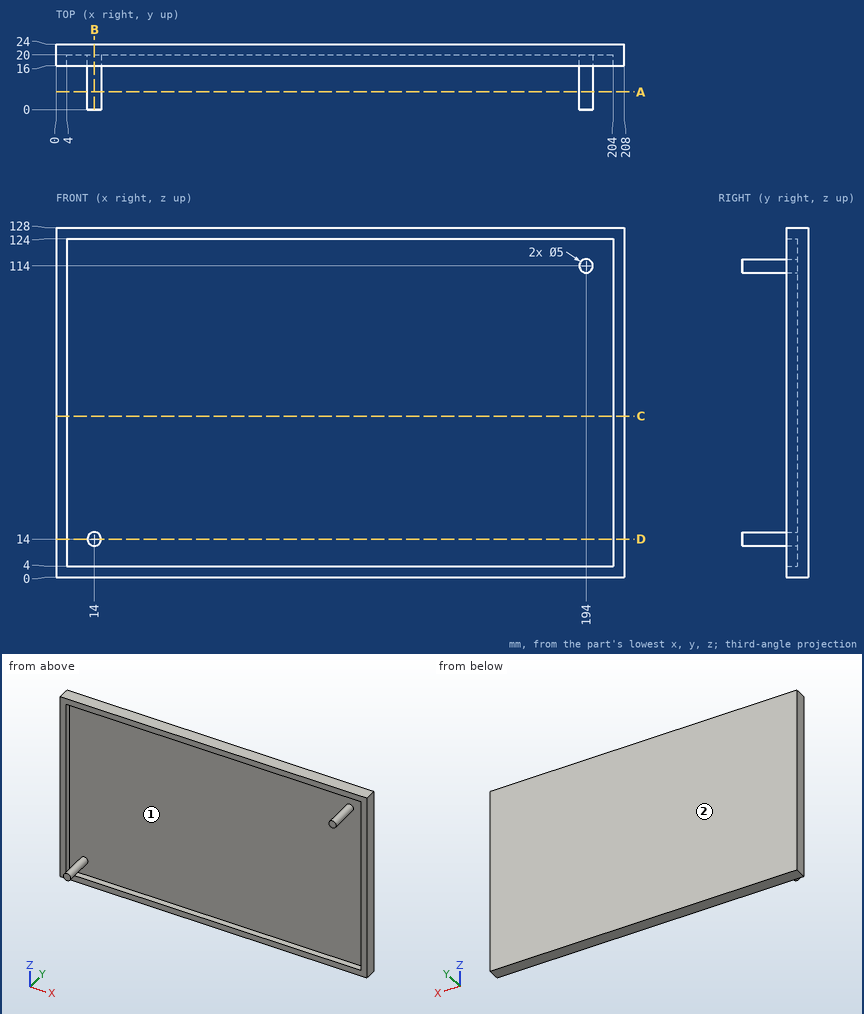
Source: three-view drawing plus pictorial views. Frame: mm from the lowest corner of the part. Give positions to 0.01 mm unless a question says otherwise; leave off trailing zeros. Loops run counter-clockwise (first coordinate to the right, second up) from the corner with the lowest first, then second, coordinate; pieces in that order, holes last. Notation, with made-up numbers: (65.5, 73.25) -> (121.5, 73.25) arc R28 cw to (121.5, 103.25) -> close; hole circle Ø4 at (8.25, 10). An arc over 180 degrees is marked (long way). Put each result on its own line as item: value. Start each with the question number.
1) Cut plane D-D (z = 14). Return loops of the section in (x, y), then the cut area to 3 significant figures.
2) Contact query for flat-ended pins moving along their axis: P1, Ø2, axis at y = 2.5, z = 115, coming from the +X side; P2, Ø6, axis at x = 97, z = 24, coming from the -Y side. Output: stop coordinate, or through.
3) Cut plane A-A (y = 6.5). Return loops of the section in (x, z).
4) Cut plane B-B (x = 14). Return loops of the section in (y, z), then the cut area to 3 significant figures.
5) Draft query along X for the marked faces 1 and 2. Return one class per face: released by +X, released by -X, zero draft, split by the parting line, or undercut.
6) Cut plane C-C (z = 59). Return loops of the section in (x, y).
7) Material intervals for probe 1 along Z at (x, y) = (43, 19.75); probe 2 along X at (y, z) = (19.5, 74.5); probe 3 along Y at (x, z) = (79.5, 79), sorted ascending.
Results are:
1. outline: (0, 16) -> (4, 16) -> (4, 20) -> (11.5, 20) -> (11.5, 0) -> (16.5, 0) -> (16.5, 20) -> (204, 20) -> (204, 16) -> (208, 16) -> (208, 24) -> (0, 24) -> close
1. area: 964 mm2
2. P1: stops at x = 196.5
2. P2: stops at y = 20
3. outline: circle Ø5 at (14, 14); circle Ø5 at (194, 114)
4. outline: (0, 11.5) -> (20, 11.5) -> (20, 4) -> (16, 4) -> (16, 0) -> (24, 0) -> (24, 128) -> (16, 128) -> (16, 124) -> (20, 124) -> (20, 16.5) -> (0, 16.5) -> close
4. area: 644 mm2
5. face 1: undercut
5. face 2: zero draft
6. outline: (0, 16) -> (4, 16) -> (4, 20) -> (204, 20) -> (204, 16) -> (208, 16) -> (208, 24) -> (0, 24) -> close
7. probe 1: z = 0 to 4, 124 to 128
7. probe 2: x = 0 to 4, 204 to 208
7. probe 3: y = 20 to 24
